Autodesk Inventor part; units mm, degrees
ref_plane "YZ Plane" through (0, 0, 0) normal (1, 0, 0) x (0, 1, 0)
ref_plane "XZ Plane" through (0, 0, 0) normal (0, 1, 0) x (-1, 0, 0)
ref_plane "XY Plane" through (0, 0, 0) normal (0, 0, 1) x (1, 0, 0)
sketch "Sketch1" plane through (0, 0, 0) normal (0, 0, 1) x (1, 0, 0)
  arc A0 (17.6188, 35.9553) -> (15.4359, 37.7539) centre (15.6281, 35.7632) ccw
  line L0 (15.4359, 37.7539) -> (-27.3652, 33.6227)
  arc A1 (-27.3652, 33.6227) -> (-29.1638, 31.4398) centre (-27.173, 31.6319) ccw
  line L1 (-29.1638, 31.4398) -> (-25.5552, -5.9466)
  arc A2 (-25.5552, -5.9466) -> (-25.0095, -6.3962) centre (-25.0575, -5.8985) ccw
  line L2 (-25.0095, -6.3962) -> (20.7777, -1.9768)
  arc A3 (20.7777, -1.9768) -> (21.2274, -1.4311) centre (20.7297, -1.4791) ccw
  line L3 (21.2274, -1.4311) -> (17.6188, 35.9553)
  circle A4 centre (-19.4703, 14.2799) radius 4.75
  circle A5 centre (11.3863, 17.2582) radius 4.75
  circle A6 centre (-18.3261, 2.3283) radius 1.25
  circle A7 centre (10.2334, 29.2027) radius 1.25
  circle A8 centre (-20.6232, 26.2244) radius 1.25
  circle A9 centre (12.5491, 5.3084) radius 1.25
  circle A10 centre (-18.3261, 2.3283) radius 1.5
  circle A11 centre (12.5491, 5.3084) radius 1.5
  circle A12 centre (10.2334, 29.2027) radius 1.5
  circle A13 centre (-20.6232, 26.2244) radius 1.5
  point P0 (0, 0)
  dimension "d0" = 3
  dimension "d1" = 3
  dimension "d3" = 3
  dimension "d6" = 3
extrude "Extrusion1" add sketch "Sketch1" along normal blind 19.05 contours L3 A3 L2 A2 L1 A1 L0 A0
properties part number "Head Spacer Plate"
Geometry check sheet. Reference: the model listing, model coordinates, mm. Give positions to 0.01 mm unless a question says otherwise; leave off trailing zeros. Order: outer loops, then holes, each group sorted by start corner. A loop starts at its lowest first (then second) coordinate and runs counter-clockwise, first axis right, second up.
1. Section check A-A, the plane y = 1.5. Enter the section's corners in (x, z).
2. Section check D-D, the plane y = 21. Enter the section's corners in (x, z).
3. Thickness scan on L1, parallel to Y at x = 10.5, z = 13.5; L2, parallel to Y at x = -21, z = 4.25; L3, parallel to Y at x = 8, z = 6. Record the ranges inside material, lowest first.
4. Section check C-C, the plane x = -17.5. Enter the section's corners in (y, z).
5. Section check B-B, the plane z = 10. Enter the section's corners in (x, y).
6. Release check for a two-part mould opening along X. For faces 1 (the face through (-4, 16, 19.05)), 2 (the face through (-28.73, 32.89, 9.39)), 3 (the face through (10.038, 27.715, 9.392)) record: pulls with the +X half, pulls with the -X half, needs draft (parallel to the pull), parting line crosses it, or undercut.
7. Gauge pin test, flat ends, axial feed: pin 1 Ø15 at (x, y) = (-19.47, 14.28) entering from -Z; pin 2 Ø1.8 at (x, y) = (-20.62, 26.22) entering from -Z; pin 3 Ø4 at (y, z) = (10, 3) entering from +X; pin 4 Ø2 at (y, z) = (8, 15) entering from -X. Record the tip position at first contact, or that the pin passes through.
Values follow:
1. outline: (-26.27, 0) - (-19.58, 0) - (-19.58, 19.05) - (-26.27, 19.05) - close; (-17.08, 0) - (20.94, 0) - (20.94, 19.05) - (-17.08, 19.05) - close
2. outline: (-28.16, 0) - (8.46, 0) - (8.46, 19.05) - (-28.16, 19.05) - close; (14.31, 0) - (19.06, 0) - (19.06, 19.05) - (14.31, 19.05) - close
3. L1: y = -2.97 to 12.59, 21.92 to 27.73, 30.68 to 37.28
3. L2: y = -6.01 to 9.78, 18.78 to 24.77, 27.68 to 34.24
3. L3: y = -3.21 to 13.93, 20.59 to 37.04
4. outline: (-5.67, 0) - (1.08, 0) - (1.08, 19.05) - (-5.67, 19.05) - close; (3.58, 0) - (9.96, 0) - (9.96, 19.05) - (3.58, 19.05) - close; (18.6, 0) - (34.57, 0) - (34.57, 19.05) - (18.6, 19.05) - close
5. outline: (-29.16, 31.44) - (-25.56, -5.95) arc R0.5 ccw to (-25.01, -6.4) - (20.78, -1.98) arc R0.5 ccw to (21.23, -1.43) - (17.62, 35.96) arc R2 ccw to (15.44, 37.75) - (-27.37, 33.62) arc R2 ccw to start; hole circle Ø9.5 at (-19.47, 14.28); hole circle Ø3 at (-20.62, 26.22); hole circle Ø3 at (-18.33, 2.33); hole circle Ø9.5 at (11.39, 17.26); hole circle Ø3 at (10.23, 29.2); hole circle Ø3 at (12.55, 5.31)
6. face 1: needs draft
6. face 2: pulls with the -X half
6. face 3: undercut
7. pin 1: stops at z = 0
7. pin 2: passes through
7. pin 3: stops at x = 20.32
7. pin 4: stops at x = -27
